Part print with two shaded views. Sizes in mm from the minimum x, y, z corner. Coordinates: 2 decimals unless noted, no trailing zeros. Write each loop counter-clockwise with the first axis right and the second up, starting at its lowest first coordinate (ties: lowest second). Pieces come first, ordered by that corner, then holes. Notation, with made-up numbers: (64.5, 85.25) - (83.5, 85.25) arc R19 cw to (83.5, 92.25) - close; hole circle Ø7 at (76.25, -1.5). An arc over 180 degrees is marked (long way). Answer in a Markdown table with one row per item. Add a question column.
Q1. Drill centre lines: line 1 along Z through (x, y) = (25, 37.5); line 2 along X through (y, z) = (16, 45) (1 decimal); line 3 along X through (y, z) = (13.5, 27). Where is each one in solid material? Low to high. Write a range as from..to.
Q2. Band-saw the part on B-B (z = 35). List the corners of the cut face in (x, y) (1 decimal).
Q3. Pin check, flat tips, straight feed: pin 1 (3 mm diameter, centred on y = 16.5, z = 49, fed in from -X) (1 decimal); pin 2 (10 mm diameter, centred on x = 24.5, y = 50, fed in from +Z); pin 3 (12 mm diameter, centred on y = 19.5, z = 14, fed in from -X) (1 decimal). Stop position of each tip, or through.
Q4. Band-saw the part on A-A (x = 28.5). List the corners of the cut face in (y, z).
Q5. Band-saw the part on C-C (y = 42). List the corners of the cut face in (x, z).
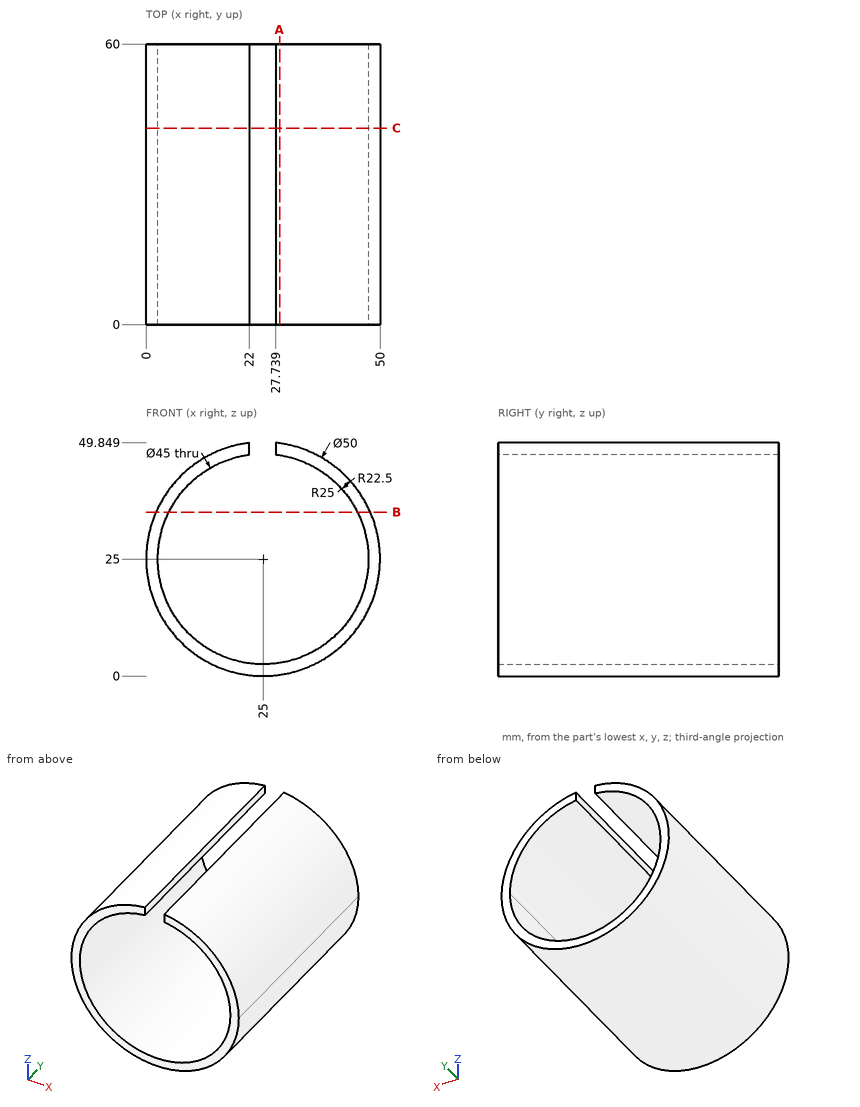
Checked values:
| question | item | result |
|---|---|---|
| 1 | line 1 | z = 0..2.5 |
| 1 | line 2 | x = 10..14.7, 35.3..40 |
| 1 | line 3 | x = 0.08..2.59, 47.41..49.92 |
| 2 | outline | (2.1, 0) - (4.8, 0) - (4.8, 60) - (2.1, 60) - close; (45.2, 0) - (47.9, 0) - (47.9, 60) - (45.2, 60) - close |
| 3 | pin 1 | stops at x = 14.1 |
| 3 | pin 2 | stops at z = 49.85 |
| 3 | pin 3 | stops at x = 0.5 |
| 4 | outline | (0, 0.25) - (60, 0.25) - (60, 2.77) - (0, 2.77) - close; (0, 47.23) - (60, 47.23) - (60, 49.75) - (0, 49.75) - close |
| 5 | outline | (22, 47.3) - (22, 49.82) arc R25 ccw (long way) to (27.74, 49.85) - (27.74, 47.33) arc R22.5 cw (long way) to start |
